Design review of the part shown in the three views and the two pictorial views. Dimensions are in mm from the part's minimum x, y and z. Coordinates: 2 decimals unless noted, no trailing zeros. Loops run counter-clockwise (first coordinate to the right, second up) from the corner with the lowest first, then second, coordinate; pieces in that order, holes last. Notation, with made-up numbers: (-35, -17.75) -> (5, -17.75) arc R9 ccw to (5, -12.75) -> close; hole circle Ø3 at (52.5, 10). An arc over 180 degrees is marked (long way). One line per item, written item: value.
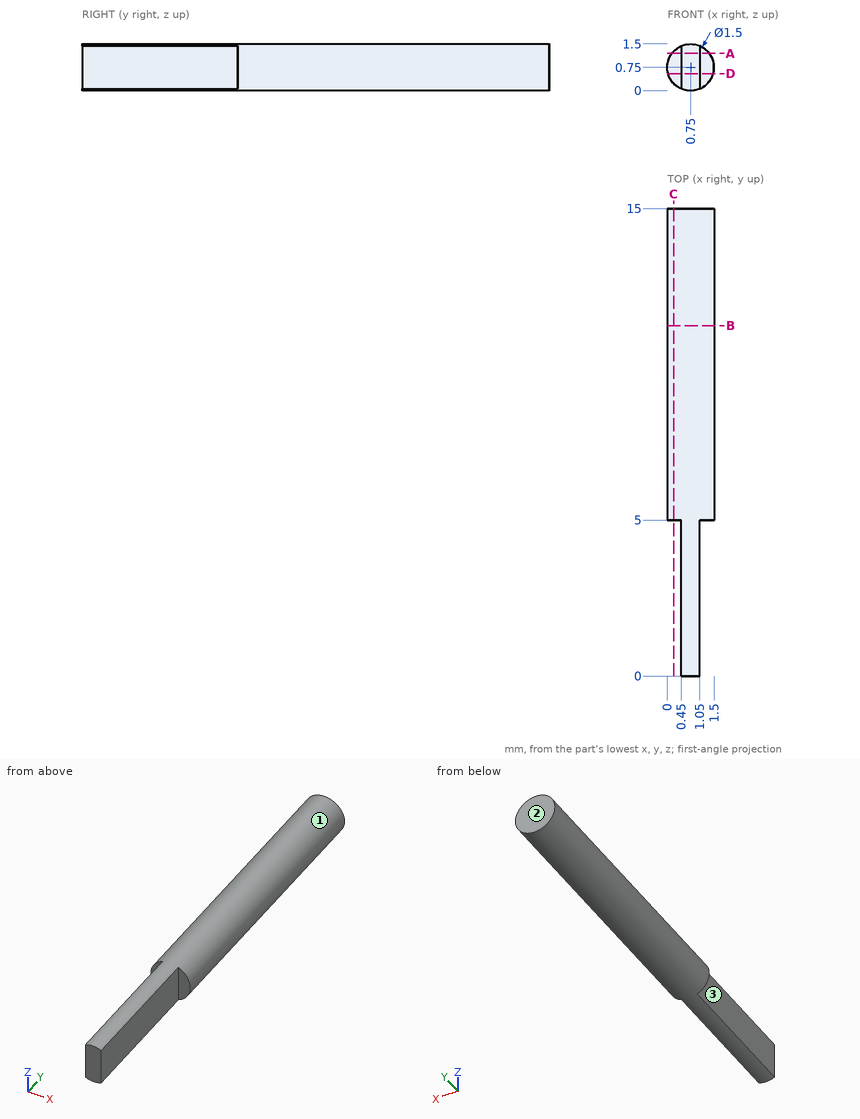
1. The part is to be moulded in two halves that separate along X. For the marked faces 1, 2 and 3, say which applies: pulls with the +X half, pulls with the -X half, needs draft (parallel to the pull), parting line crosses it, or undercut.
Return value:
face 1: parting line crosses it
face 2: needs draft
face 3: pulls with the -X half
2. Insertion check: pin 1 Ø0.7 at (y, z) = (2, 1) entering from +X. The pin has a flat end and moves straight along its axis. Give the tip position at first contact, or say it passes through.
Return value:
pin 1: stops at x = 1.05
3. Take a section at C-C, the plane x = 0.2. Give the boundary of the cut face in (y, z).
Return value:
outline: (5, 0.24) -> (15, 0.24) -> (15, 1.26) -> (5, 1.26) -> close
4. Take a section at A-A, the plane z = 1.2. Give the boundary of the cut face in (x, y), and give its area (3 significant figures).
Return value:
outline: (0.15, 5) -> (0.45, 5) -> (0.45, 0) -> (1.05, 0) -> (1.05, 5) -> (1.35, 5) -> (1.35, 15) -> (0.15, 15) -> close
area: 15.0 mm2
5. Take a section at D-D, the plane z = 0.55. Give the boundary of the cut face in (x, y), and give its area (3 significant figures).
Return value:
outline: (0.03, 5) -> (0.45, 5) -> (0.45, 0) -> (1.05, 0) -> (1.05, 5) -> (1.47, 5) -> (1.47, 15) -> (0.03, 15) -> close
area: 17.5 mm2
6. To check wall thickness, follow probe 1 along X at (y, z) = (3.5, 1.35); probe 2 along Y at (x, z) = (0.4, 0.25); probe 3 along X at (y, z) = (8, 0.8). State the ranges of each line that lie inside material, in increasing order. Write a range as from..to.
Return value:
probe 1: x = 0.45..1.05
probe 2: y = 5..15
probe 3: x = 0..1.5
7. Take a section at B-B, the plane y = 11.25. Give the boundary of the cut face in (x, z), and give its area (3 significant figures).
Return value:
outline: circle Ø1.5 at (0.75, 0.75)
area: 1.77 mm2
